```python
from build123d import *

# Parameters (mm, degrees)
SKETCH_1_R          = 2.5
EXTRUDE_1_DEPTH     = 7
SKETCH_1_5_R        = 14
SKETCH_1_5_R_2      = 9
EXTRUDE_3_DEPTH     = 30
SKETCH_1_6_R        = 9
CUT_EXTRUDE_2_DEPTH = 7
CHAMFER_1_SIZE      = 4
CHAMFER_1_SIZE2     = 2.309401077


with BuildPart() as part:
    # Sketch 1 → Extrude 1 (new body)
    with BuildSketch(Plane.XY):
        with BuildLine():
            Line((-24.5, 3.122498999), (-11.454897552, 13.884715412))
            ThreePointArc((-11.454897552, 13.884715412), (0, 18), (11.454897552, 13.884715412))
            Line((11.454897552, 13.884715412), (24.5, 3.122498999))
            ThreePointArc((24.5, 3.122498999), (26, 0), (24.5, -3.122498999))
            Line((24.5, -3.122498999), (11.454897552, -13.884715412))
            ThreePointArc((11.454897552, -13.884715412), (0, -18), (-11.454897552, -13.884715412))
            Line((-11.454897552, -13.884715412), (-24.5, -3.122498999))
            ThreePointArc((-24.5, -3.122498999), (-26, 0), (-24.5, 3.122498999))
        make_face()
        with Locations((-22, 0)):
            Circle(SKETCH_1_R, mode=Mode.SUBTRACT)
        with Locations((22, 0)):
            Circle(SKETCH_1_R, mode=Mode.SUBTRACT)
    extrude(amount=EXTRUDE_1_DEPTH)

    # Sketch 1_5 → Extrude 3 (add)
    with BuildSketch(Plane.XY):
        Circle(SKETCH_1_5_R)
        Circle(SKETCH_1_5_R_2, mode=Mode.SUBTRACT)
    extrude(amount=EXTRUDE_3_DEPTH)

    # Sketch 1_6 → Cut-Extrude 2 (cut)
    with BuildSketch(Plane.XY):
        Circle(SKETCH_1_6_R)
    extrude(amount=CUT_EXTRUDE_2_DEPTH, mode=Mode.SUBTRACT)

    # Chamfer 1
    chamfer_1_edges = [part.edges().sort_by_distance(p)[0] for p in [
        (-9, 0, 30),
    ]]
    chamfer_1_side = [part.faces().sort_by_distance(p)[0] for p in [
        (-13.604020203, 0, 30),
    ]]
    chamfer(chamfer_1_edges, length=CHAMFER_1_SIZE, length2=CHAMFER_1_SIZE2, reference=chamfer_1_side[0])


solid = part.part
```
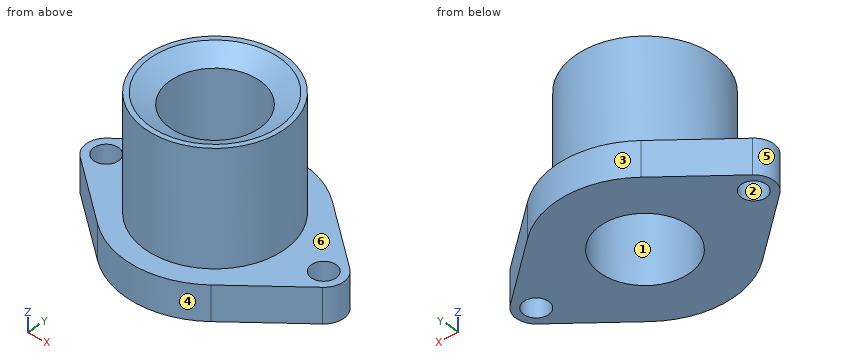
Build history of the part. All positions in model axes, mm. Face numbers are marked on the shaded views. A direction names the side the tool comes from. Coordinates: 2 decimals unless noted, no trailing zeros. Order: outer loops, then holes, each group sorted by start corner. A loop starts at its lowest first (then second) coordinate and runs counter-clockwise, first axis right, second up.
Item 1: Drill centre lines: L1, parallel to Y at x = 0.5, z = 22.5; L2, parallel to Z at x = 21.5, y = 2.5; L3, parallel to X at y = 1.5, z = 5.5. Where is each one in solid material? Low to high.
Filled in:
L1: y = -13.99 to -8.99, 8.99 to 13.99
L2: z = 0 to 7
L3: x = -25.71 to -24, -20 to -8.87, 8.87 to 20, 24 to 25.71
Item 2: Mould opens along Y. For the marked faces 1, 2, 3 and 4 say: released by +Y, released by -Y, zero draft, split by the parting line, or undercut.
Filled in:
face 1: undercut
face 2: undercut
face 3: released by +Y
face 4: released by -Y
Item 3: Saw through at A-A on x = 0. List the corners of the cut face in (y, z).
Filled in:
outline: (-18, 0) - (-9, 0) - (-9, 27.69) - (-13, 30) - (-14, 30) - (-14, 7) - (-18, 7) - close; (9, 0) - (18, 0) - (18, 7) - (14, 7) - (14, 30) - (13, 30) - (9, 27.69) - close
Item 4: Saw through at B-B on z = 26.5. List the corners of the cut face in (x, y), then the cut area to 3 significant figures.
Filled in:
outline: circle Ø28 at (0, 0); hole circle Ø18 at (0, 0)
area: 361 mm2
Item 5: Drop flat-ended pins along their axis: pin 1 Ø6.5 at (x, y) = (22, 0) entering from +Z; pin 2 Ø11 at (x, y) = (0, 0) entering from -Z; pin 3 Ø1.5 at (x, y) = (-1.5, 12) entering from +Z; pin 4 Ø5 at (y, z) = (-9.5, 24.5) entering from +X. Give the stop position or say it passes through.
Filled in:
pin 1: stops at z = 7
pin 2: passes through
pin 3: stops at z = 29.91
pin 4: stops at x = 12.12
Item 6: Tool access for the marked faces 5 and 6: list every direction of +Z, -Z, +X, -X, +Y, -Y with a clear straight run to the whole face (end or side of a thin tool).
Filled in:
face 5: +Z, -Z, -X
face 6: +Z
Item 7: Saw through at D-D on x = 22.5. List the corners of the cut face in (y, z), then the cut area to 3 significant figures.
Filled in:
outline: (-4.77, 0) - (-2.45, 0) - (-2.45, 7) - (-4.77, 7) - close; (2.45, 0) - (4.77, 0) - (4.77, 7) - (2.45, 7) - close
area: 32.5 mm2
Item 8: Saw through at C-C on x = -22. List the corners of the cut face in (y, z) (3 decimals).
Filled in:
outline: (-5.185, 0) - (-2.5, 0) - (-2.5, 7) - (-5.185, 7) - close; (2.5, 0) - (5.185, 0) - (5.185, 7) - (2.5, 7) - close
